Geometry: see drawing. Coordinates: mm, zero at the bounding-box minimum. A direction names the side the tool comes from. Give positions to 0.01 mm unless a question says otherwise; leave off trailing zeros. Order: outer loops, then holes, each group sorted by start corner. A loop starts at its lowest first (then second) coordinate and runs counter-clockwise, first axis right, second up. Notation, with made-up numbers: (60, -4) - (81, -4) arc R25 cw to (81, 20) - close; hole circle Ø3 at (81, -3). An arc over 180 degrees is marked (long way). One line per question, with ' | ' between items. Start each with the question number.
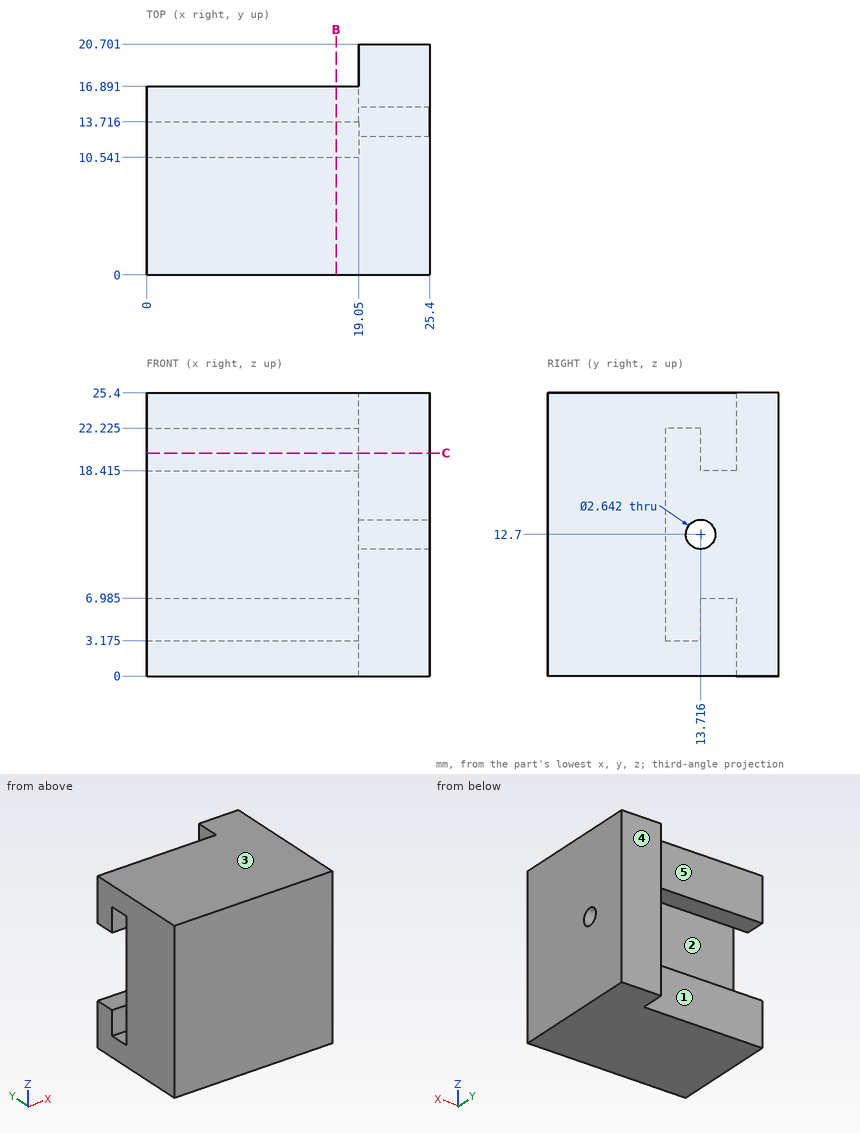
(1) Cut plane C-C, the plane z = 20. Return the cut outline in (x, y), plus the area to 3 significant figures.
(2) Access query for the marked faces 4 and 5. Directions: +Z, -Z, +X, -X, +Y, -Y. A direction counts if a zero-diameter tool reaches every point of the face in a straight line with its end or side. Return the directions, or none.
(3) Contact query for flat-ended pins moving along their axis: P1, Ø4, axis at y = 13.716, z = 12.7, coming from the +X side; P2, Ø5.5, axis at x = 12, z = 21.5, coming from the +Y side. Output: stop coordinate, or through.
(4) Material intervals for line 1 along Z through (x, y) = (9, 14.5) (1 decimal); line 2 along Y through (x, z) = (22, 12.7) (1 decimal); line 3 along Y through (x, z) = (1.25, 20.75), sorted ascending. Write a range as from..to.
(5) Pull-direction query (Z, two-part tool) for the marked faces 1, 2 and 3; classes: +Z half, -Z half, draft (parallel to the pull), parting line (faces both ways), or undercut.
(6) Cut plane B-B, the plane x = 17. Return the cut outline in (y, z) (1 decimal).
Results are:
1) outline: (0, 0) - (25.4, 0) - (25.4, 20.7) - (19.05, 20.7) - (19.05, 16.89) - (0, 16.89) - (0, 13.72) - (19.05, 13.72) - (19.05, 10.54) - (0, 10.54) - close | area: 393 mm2
2) face 4: +Z, -Z, +X, -X, +Y | face 5: +Z, -Z, -X, +Y
3) P1: x = 25.4 | P2: y = 16.89
4) line 1: 0..7, 18.4..25.4 | line 2: 0..12.4, 15..20.7 | line 3: 0..10.54, 13.72..16.89
5) face 1: draft | face 2: undercut | face 3: +Z half
6) outline: (0, 0) - (16.9, 0) - (16.9, 7) - (13.7, 7) - (13.7, 3.2) - (10.5, 3.2) - (10.5, 22.2) - (13.7, 22.2) - (13.7, 18.4) - (16.9, 18.4) - (16.9, 25.4) - (0, 25.4) - close
